The listing builds one solid part. Answer for the finished solid, in the listing's coordinates (mm). A direction names the side the tool comes from. Give positions to 0.01 mm unless a question says otherwise; leave off trailing zeros. Order: outer loops, then holes, each group sorted by start corner. A loop starts at its lowest first (then second) coordinate and runs counter-clockwise, first axis right, second up. Notation, with made-up numbers: (81.25, 77.5) - (92.25, 77.5) arc R6 ccw to (92.25, 82.5) - close; hole circle Ø10 at (-11.5, -27.5). An arc over 180 degrees is marked (long way). Answer as a JSON object with one key per item and string values. Group by question number.
Q1. A cutting plane is placed at B-B, the plane z = 13.5. Give the vertices of the cut face in (x, y).
Q2. The mould has two halves that part along Y. Classify faces 4 (the face through (28.2, 5.9, 5)), 5 (the face through (26.924, -44, 10)), 6 (the face through (28.212, 6.169, 19.176)): released by +Y, released by -Y, zero draft, split by the parting line, or undercut.
Q3. A cutting plane is placed at A-A, the plane y = -44.45. Give the vertices of the cut face in (x, z).
Q4. A cutting plane is placed at C-C, the plane x = 7. Give the vertices of the cut face in (y, z), and give its area (3 significant figures).
Q5. For faces 1 (the face through (13, -40.64, 10)), 2 (the face through (33, 0, 10)), 3 (the face through (13, 0, 10)), determine the directions among +Z, -Z, +X, -X, +Y, -Y from which every point of the face is accessible in a straight line to the end or side of a thin tool.
Q6. Consider line 1 (Y direction, x = 27.5, z = 14.5); line 2 (Y direction, x = 9, z = 11.75); line 3 (X direction, y = -41.5, z = 4.5). Determine where each line is inside the solid, lowest interval first.
Q7. Given pin 1 (5.5 mm diameter, centred on y = -44.45, z = 14.9, fed in from +X); pin 2 (4 mm diameter, centred on x = 24, z = 10.5, fed in from +Y); pin 3 (10 mm diameter, centred on x = 8, z = 2.5, fed in from -Y); pin 4 (4 mm diameter, centred on y = -44.45, z = 4.74, fed in from +X), each flat-ended and moving along its own axis, determine where each tip first touches the part or whether it passes through.
Q8. A cutting plane is placed at D-D, the plane z = 8.75. Give the vertices of the cut face in (x, y).
Autodesk Inventor part; units mm, degrees
ref_plane "YZ Plane" through (0, 0, 0) normal (1, 0, 0) x (0, 1, 0)
ref_plane "XZ Plane" through (0, 0, 0) normal (0, 1, 0) x (-1, 0, 0)
ref_plane "XY Plane" through (0, 0, 0) normal (0, 0, 1) x (1, 0, 0)
sketch "Sketch1" plane through (0, 0, 0) normal (0, 0, 1) x (1, 0, 0)
  line L0 (0, 0) -> (0, -40.64)
  line L1 (0, -40.64) -> (26.924, -40.64)
  line L2 (0, 0) -> (26.924, 0)
  line L3 (26.924, -40.64) -> (26.924, -47.244)
  line L4 (26.924, -47.244) -> (29.464, -47.244)
  line L5 (29.464, -47.244) -> (29.464, -40.64)
  line L6 (26.924, 0) -> (26.924, 6.604)
  line L7 (26.924, 6.604) -> (29.464, 6.604)
  line L8 (29.464, 6.604) -> (29.464, 0)
  line L9 (29.464, 0) -> (37.084, 0)
  line L10 (29.464, -40.64) -> (37.084, -40.64)
  line L11 (37.084, 0) -> (37.084, -40.64)
  dimension "d0" = 40.64
  dimension "d4" = 6.604
  dimension "d45" = 2.54
  dimension "d46" = 26.924
  dimension "d47" = 7.62
extrude "Extrusion8" add sketch "Sketch1" along normal blind 19.6342
sketch "Sketch8" plane through (37.084, -40.64, 0) normal (1, 0, 0) x (0, 0, -1)
  line L0 (0, 0) -> (0, 40.64)
  line L1 (0, 40.64) -> (-19.6342, 40.64)
  line L2 (-19.6342, 0) -> (-19.6342, 40.64)
  line L3 (0, 0) -> (-19.6342, 0)
  circle A0 centre (-9.8171, 30.861) radius 6.477
  dimension "d50" = 12.954
  dimension "d51" = 9.779
extrude "Extrusion9" add sketch "Sketch8" along normal blind 1.778 contours A0
sketch "Sketch9" plane through (29.464, 0, 0) normal (1, 0, 0) x (0, 0, -1)
  circle A0 centre (-14.8971, 3.81) radius 2.1082
  line L0 (0, 6.604) -> (-19.6342, 6.604)
  line L1 (-9.8171, 6.604) -> (-9.8171, 8.0872)
  line L2 (0, 0) -> (-19.6342, 0)
  circle A1 centre (-4.7371, 3.81) radius 2.1082
  line L3 (0, 0) -> (0, -40.64)
  line L4 (0, -20.32) -> (8.7495, -20.32)
  circle A2 centre (-14.8971, -44.45) radius 2.1082
  circle A3 centre (-4.7371, -44.45) radius 2.1082
  dimension "d54" = 4.2164
  dimension "d55" = 5.08
  dimension "d56" = 3.81
extrude "Extrusion10" cut sketch "Sketch9" against normal through all
fillet "Fillet1" radius 1.524 4 edges at (28.194, 6.604, 19.6342) (28.194, 6.604, 0) (28.194, -47.244, 19.6342) (28.194, -47.244, 0)
properties part number "Servo" material "ABS Plastic"
Reply:
{
 "1": {"outline": "(0, -40.64) - (26.92, -40.64) - (26.92, -42.87) - (29.46, -42.87) - (29.46, -40.64) - (37.08, -40.64) - (37.08, -15.11) - (38.86, -15.11) - (38.86, -4.45) - (37.08, -4.45) - (37.08, 0) - (29.46, 0) - (29.46, 2.23) - (26.92, 2.23) - (26.92, 0) - (0, 0) - close; (26.92, -47.24) - (29.46, -47.24) - (29.46, -46.03) - (26.92, -46.03) - close; (26.92, 5.39) - (29.46, 5.39) - (29.46, 6.6) - (26.92, 6.6) - close"},
 "2": {"face 4": "undercut", "face 5": "zero draft", "face 6": "released by +Y"},
 "3": {"outline": "(26.92, 0) - (29.46, 0) - (29.46, 2.63) - (26.92, 2.63) - close; (26.92, 6.85) - (29.46, 6.85) - (29.46, 12.79) - (26.92, 12.79) - close; (26.92, 17.01) - (29.46, 17.01) - (29.46, 19.63) - (26.92, 19.63) - close"},
 "4": {"outline": "(-40.64, 0) - (0, 0) - (0, 19.63) - (-40.64, 19.63) - close", "area": "798 mm^2"},
 "5": {"face 1": "+Z, -Z, -X, -Y", "face 2": "+Z, -Z, +X, +Y", "face 3": "+Z, -Z, -X, +Y"},
 "6": {"line 1": "y = -47.24 to -46.52, -42.38 to 1.74, 5.88 to 6.6", "line 2": "y = -40.64 to 0", "line 3": "x = 26.92 to 29.46"},
 "7": {"pin 1": "stops at x = 29.46", "pin 2": "stops at y = 0", "pin 3": "stops at y = -40.64", "pin 4": "passes through"},
 "8": {"outline": "(0, -40.64) - (26.92, -40.64) - (26.92, -47.24) - (29.46, -47.24) - (29.46, -40.64) - (37.08, -40.64) - (37.08, -16.17) - (38.86, -16.17) - (38.86, -3.39) - (37.08, -3.39) - (37.08, 0) - (29.46, 0) - (29.46, 6.6) - (26.92, 6.6) - (26.92, 0) - (0, 0) - close"}
}
